```python
from build123d import *

# Parameters (mm, degrees)
SKETCH_1_W          = 42.3
SKETCH_1_H          = 42.3
EXTRUDE_1_DEPTH     = 2
SKETCH_2_R          = 1.6
CUT_EXTRUDE_1_DEPTH = 3
SKETCH_3_R          = 7.5
EXTRUDE_2_DEPTH     = 10
SKETCH_4_R          = 2.525
CUT_EXTRUDE_3_DEPTH = 13
FILLET_1_R          = 5
CUT_EXTRUDE_4_REACH = 30.65
SKETCH_5_R          = 2


with BuildPart() as part:
    # 草图1 → 凸台-拉伸1 (new body)
    with BuildSketch(Plane(origin=(0, 0, 0), x_dir=(1, 0, 0), z_dir=(0, 1, 0))):
        Rectangle(SKETCH_1_W, SKETCH_1_H)
    extrude(amount=EXTRUDE_1_DEPTH)

    # 草图2 → 切除-拉伸1 (cut, through all)
    with BuildSketch(Plane(origin=(0, 2, 0), x_dir=(1, 0, 0), z_dir=(0, 1, 0))):
        with Locations((-15.5, 15.5)):
            Circle(SKETCH_2_R)
        with Locations((15.5, 15.5)):
            Circle(SKETCH_2_R)
        with Locations((15.5, -15.5)):
            Circle(SKETCH_2_R)
        with Locations((-15.5, -15.5)):
            Circle(SKETCH_2_R)
    extrude(amount=-CUT_EXTRUDE_1_DEPTH, mode=Mode.SUBTRACT)

    # 草图3 → 凸台-拉伸2 (add)
    with BuildSketch(Plane(origin=(0, 2, 0), x_dir=(1, 0, 0), z_dir=(0, 1, 0))):
        Circle(SKETCH_3_R)
    extrude(amount=EXTRUDE_2_DEPTH)

    # 草图4 → 切除-拉伸3 (cut, through all)
    with BuildSketch(Plane(origin=(0, 12, 0), x_dir=(1, 0, 0), z_dir=(0, 1, 0))):
        Circle(SKETCH_4_R)
    extrude(amount=-CUT_EXTRUDE_3_DEPTH, mode=Mode.SUBTRACT)

    # 圆角1
    fillet_1_edges = [part.edges().sort_by_distance(p)[0] for p in [
        (21.15, 1, 21.15),
        (-21.15, 1, 21.15),
        (-21.15, 1, -21.15),
        (21.15, 1, -21.15),
    ]]
    fillet(fillet_1_edges, radius=FILLET_1_R)

    # 草图5 → 切除-拉伸4 (cut, up to next)
    with BuildSketch(Plane.XY.offset(7.5), mode=Mode.PRIVATE) as cut_extrude_4_sk1:
        with Locations((0, 7)):
            Circle(SKETCH_5_R)
    cut_extrude_4_tool1 = extrude(cut_extrude_4_sk1.sketch, amount=-CUT_EXTRUDE_4_REACH, mode=Mode.PRIVATE) & part.part
    add(cut_extrude_4_tool1.solids().sort_by_distance((0, 7, 7.5))[0], mode=Mode.SUBTRACT)


solid = part.part
```
Geometry check sheet. Reference: the model listing, model coordinates, mm. A direction names the side the tool comes from. Coordinates: 2 decimals unless noted, no trailing zeros. Write each loop counter-clockwise with the first axis right and the second up, starting at its lowest first coordinate (ties: lowest second). Pieces come first, ordered by that corner, then holes. Notation, with made-up numbers: M 46.5,37 L 74.5,37 A32 cw 74.5,69 Z; hole C -25,29 d7. An arc over 180 degrees is marked long. Answer as a JSON object with one key per item and string values.
1. Section check B-B, the plane z = 0. Enter the section's corners in (x, y) (3 decimals), plus the area to 3 significant figures.
Answers below:
{"outline": "M -21.15,0 L -2.525,0 L -2.525,12 L -7.5,12 L -7.5,2 L -21.15,2 Z; M 2.525,0 L 21.15,0 L 21.15,2 L 7.5,2 L 7.5,12 L 2.525,12 Z", "area": "174 mm²"}
2. Scan lines: L1, parallel to Z at x = -15.5, y = 1.5; L2, parallel to X at y = 8, z = 0 (3 decimals). Record each from-to range of solid material in increasing order.
Answers below:
{"L1": "z = -21.15 to -17.1, -13.9 to 13.9, 17.1 to 21.15", "L2": "x = -7.5 to -2.525, 2.525 to 7.5"}
3. Go/stop test with flat-tipped pins: pin 1 Ø5 at (x, z) = (15.5, -15.5) entering from +Y; pin 2 Ø2 at (x, y) = (-2.5, 7) entering from +Z; pin 3 Ø1.5 at (y, z) = (4.5, -2) entering from +X. Record where each tip stops, or that it passes through.
Answers below:
{"pin 1": "stops at y = 2", "pin 2": "stops at z = 7.27", "pin 3": "stops at x = 7.4"}
4. Draft check along Y on faces 1 (the cylindrical face through (1.908, 7.601, 4.563)), 2 (the cylindrical face through (19.65, 1.01, 19.72)), 3 (the flat face through (0, 0, 4)), 4 (the flat face through (3, 12, 0)). Enter one of: released by +Y, released by -Y, zero draft, split by the parting line, or undercut.
Answers below:
{"face 1": "undercut", "face 2": "zero draft", "face 3": "released by -Y", "face 4": "released by +Y"}
5. Tool access check on faces 5 (the cylindrical face through (-19.72, 1.01, -19.65)), 6 (the flat face through (9, 2, 0)). Record the directions out of +Z, -Z, +X, -X, +Y, -Y that give a thin tool (end or side, any length) a straight path to the whole face; none if there is none.
Answers below:
{"face 5": "-Z, -X, +Y, -Y", "face 6": "+Y"}
6. Section check C-C, the plane y = 4.25. Enter the section's corners in (x, z) (3 decimals), plus the area to 3 significant figures.
Answers below:
{"outline": "C 0,0 d15; hole C 0,0 d5.05", "area": "157 mm²"}
7. Section check D-D, the plane z = -12.5. Enter the section's corners in (x, y).
Answers below:
{"outline": "M -21.15,0 L 21.15,0 L 21.15,2 L -21.15,2 Z"}
8. Section check A-A, the plane x = 15.5. Enter the section's corners in (y, z), plus the area to 3 significant figures.
Answers below:
{"outline": "M 0,-21.15 L 2,-21.15 L 2,-17.1 L 0,-17.1 Z; M 0,-13.9 L 2,-13.9 L 2,13.9 L 0,13.9 Z; M 0,17.1 L 2,17.1 L 2,21.15 L 0,21.15 Z", "area": "71.8 mm²"}
